Geometry: final body of the model. Coordinates: model frame, mm. A direction names the side the tool comes from. Give positions to 0.01 mm unless a question says otherwise; leave off trailing zeros. Loops run counter-clockwise (first coordinate to the right, second up) from the corner with the lowest first, then second, coordinate; pieces in that order, holes last.
```python
from build123d import *

# Parameters (mm, degrees)
F1_DEPTH = 101.6
F2_W     = 6.35
F2_H     = 1.27
F2_W_2   = 3.5404078662
F2_H_2   = 5.08
F3_DEPTH = 12.7
F4_DEPTH = 12.7


with BuildPart() as f1:
    # F0 (on Top) → F1 (new body)
    with BuildSketch(Plane.XY):
        Polygon((0, 38.1), (-30.48, 15.961895347), (-30.48, 0), (0, 0), align=None)
    extrude(amount=F1_DEPTH)

    # F2 (on face) → F3 (cut)
    with BuildSketch(Plane.YZ):
        with Locations((24.2689500645, 86.7467758033)):
            Rectangle(F2_W, F2_H)
        with Locations((24.3418384343, 75.3167758033)):
            Rectangle(F2_W, F2_H)
        with Locations((13.6419944465, 80.9715090013)):
            Rectangle(F2_W_2, F2_H_2)
        with BuildLine():
            ThreePointArc((15.4121983796, 78.4315090013), (17.9521983796, 80.9715090013), (15.4121983796, 83.5115090013))
            Line((15.4121983796, 83.5115090013), (15.4121983796, 78.4315090013))
        make_face()
    extrude(amount=-F3_DEPTH, mode=Mode.SUBTRACT)

    # F2 (on face) → F4 (cut)
    with BuildSketch(Plane.YZ):
        with Locations((24.3418384343, 26.2832241967)):
            Rectangle(F2_W, F2_H)
        with Locations((24.2689500645, 14.8532241967)):
            Rectangle(F2_W, F2_H)
        with BuildLine():
            ThreePointArc((15.4121983796, 18.0884909987), (17.9521983796, 20.6284909987), (15.4121983796, 23.1684909987))
            Line((15.4121983796, 23.1684909987), (15.4121983796, 18.0884909987))
        make_face()
        with Locations((13.6419944465, 20.6284909987)):
            Rectangle(F2_W_2, F2_H_2)
    extrude(amount=-F4_DEPTH, mode=Mode.SUBTRACT)


solid = f1.part
```
Q1. Pin query (flat end, axial travel): pin 1 Ø4 at (x, z) = (-26, 29) entering from +Y; pin 2 Ø1.4 at (x, z) = (-7.5, 75.5) entering from +Y; pin 3 Ø4 at (x, z) = (-7, 21.5) entering from +Y. Return the tip coordinate at first contact, or that it passes through.
Q2. Section query A-A, the plane x = -11. Return loops of the section in (y, z).
Q3. Section query C-C, the plane x = -27.5. Return loops of the section in (y, z).
Q4. Section query D-D, the plane x = -6.5. Return loops of the section in (y, z), and give its area (3 significant figures).
Q5. Reachability of faces 1 (the face through (-15.027, 27.186, 50.089)), 2 (the face through (-6.26, 17.95, 80.92)) from +Z, -Z, +X, -X, +Y, -Y: full face, straight path, thin tool, end or side. Return the list, or none.
Q6. Material intervals for probe 1 along Z at (x, y) = (-7, 15); probe 2 along Z at (x, y) = (-10, 21.5); probe 3 along Y at (x, z) = (-7, 79.5), sorted ascending.
Q7. Section query B-B, the plane z = 59. Return loops of the section in (x, y).
Q8. Mould query, pull axis Z, two halves, no side actions, for faces 3 (the face through (-12.7, 15, 81)), 4 (the face through (-12, 15, 0)), 5 (the face through (-12, 15, 101.6)), 6 (the face through (0, 19, 50)). Classes: +Z half, -Z half, draft (parallel to the pull), parting line (faces both ways), or undercut.
Resolved:
1. pin 1: stops at y = 20.67
1. pin 2: stops at y = 33.16
1. pin 3: stops at y = 34.47
2. outline: (0, 0) - (30.11, 0) - (30.11, 101.6) - (0, 101.6) - close; hole (11.87, 18.09) - (15.41, 18.09) arc R2.54 ccw to (15.41, 23.17) - (11.87, 23.17) - close; hole (11.87, 78.43) - (15.41, 78.43) arc R2.54 ccw to (15.41, 83.51) - (11.87, 83.51) - close; hole (21.09, 14.22) - (27.44, 14.22) - (27.44, 15.49) - (21.09, 15.49) - close; hole (21.09, 86.11) - (27.44, 86.11) - (27.44, 87.38) - (21.09, 87.38) - close; hole (21.17, 25.65) - (27.52, 25.65) - (27.52, 26.92) - (21.17, 26.92) - close; hole (21.17, 74.68) - (27.52, 74.68) - (27.52, 75.95) - (21.17, 75.95) - close
3. outline: (0, 0) - (18.13, 0) - (18.13, 101.6) - (0, 101.6) - close
4. outline: (0, 0) - (33.38, 0) - (33.38, 101.6) - (0, 101.6) - close; hole (11.87, 18.09) - (15.41, 18.09) arc R2.54 ccw to (15.41, 23.17) - (11.87, 23.17) - close; hole (11.87, 78.43) - (15.41, 78.43) arc R2.54 ccw to (15.41, 83.51) - (11.87, 83.51) - close; hole (21.09, 14.22) - (27.44, 14.22) - (27.44, 15.49) - (21.09, 15.49) - close; hole (21.09, 86.11) - (27.44, 86.11) - (27.44, 87.38) - (21.09, 87.38) - close; hole (21.17, 25.65) - (27.52, 25.65) - (27.52, 26.92) - (21.17, 26.92) - close; hole (21.17, 74.68) - (27.52, 74.68) - (27.52, 75.95) - (21.17, 75.95) - close
4. area: 3,300 mm2
5. face 1: +Z, -Z, -X, +Y
5. face 2: +X
6. probe 1: z = 0 to 18.09, 23.17 to 78.43, 83.51 to 101.6
6. probe 2: z = 0 to 14.22, 15.49 to 25.65, 26.92 to 74.68, 75.95 to 86.11, 87.38 to 101.6
6. probe 3: y = 0 to 11.87, 17.48 to 33.02
7. outline: (-30.48, 0) - (0, 0) - (0, 38.1) - (-30.48, 15.96) - close
8. face 3: undercut
8. face 4: -Z half
8. face 5: +Z half
8. face 6: draft
